Build history of the part. All positions in model axes, mm. Coordinates: 2 decimals unless noted, no trailing zeros. Write each loop counter-clockwise with the first axis right and the second up, starting at its lowest first coordinate (ties: lowest second). Pieces come first, ordered by that corner, then holes.
```python
from build123d import *

# Parameters (mm, degrees)
BASE_FLANGE1_DEPTH    = 76.2
CUT_EXTRUDE1_DEPTH    = 100.11903454
SKETCH4_R             = 8.334375
CUT_EXTRUDE2_DEPTH    = 100.669004783
FILLET1_R             = 9.525
FLAT_PATTERN1_START   = 4.7752
FLAT_PATTERN1_DEPTH   = 41.610875653
FLAT_PATTERN1_2_DEPTH = 4.7752
SKETCH6_R             = 4.9657
CUT_EXTRUDE4_DEPTH    = 89.346165933


# Read off the part's stored shape, not the designer's step: Flat-Pattern1
# Sheet-metal steps are written as plain solids
with BuildPart() as part:
    # Sketch1 → Base-Flange1 (new, symmetric)
    with BuildSketch(Plane(origin=(0, 0, 0), x_dir=(0, 0, -1), z_dir=(1, 0, 0))):
        with BuildLine():
            Line((0, 44.45), (0, 3.610410109))
            ThreePointArc((0, 3.610410109), (-0.932488229, 0.652935287), (-3.392675737, -1.234832983))
            Line((-3.392675737, -1.234832983), (-44.752861065, -16.288709326))
            Line((-44.752861065, -16.288709326), (-46.386075653, -11.801489123))
            Line((-46.386075653, -11.801489123), (-5.025890325, 3.25238722))
            ThreePointArc((-5.025890325, 3.25238722), (-4.844103071, 3.391877486), (-4.7752, 3.610410109))
            Line((-4.7752, 3.610410109), (-4.7752, 44.45))
            Line((-4.7752, 44.45), (0, 44.45))
        make_face()
    extrude(amount=BASE_FLANGE1_DEPTH, both=True)

    # Sketch3 → Cut-Extrude1 (cut, through all)
    with BuildSketch(Plane(origin=(0, -7.918276224, 35.717035898), x_dir=(1, 0, 0), z_dir=(0, -0.9396926207859093, -0.3420201433256664))):
        with BuildLine():
            Line((-76.2, -20.318857819), (-16.138866151, 7.766752504))
            ThreePointArc((-16.138866151, 7.766752504), (0, 11.353754961), (16.138866151, 7.766752504))
            Line((16.138866151, 7.766752504), (76.2, -20.318857819))
            Line((76.2, -20.318857819), (88.840930233, -20.318857819))
            Line((88.840930233, -20.318857819), (88.840930233, 63.227466393))
            Line((88.840930233, 63.227466393), (-88.840930233, 63.227466393))
            Line((-88.840930233, 63.227466393), (-88.840930233, -20.318857819))
            Line((-88.840930233, -20.318857819), (-76.2, -20.318857819))
        make_face()
    extrude(amount=CUT_EXTRUDE1_DEPTH, mode=Mode.SUBTRACT)

    # Sketch4 → Cut-Extrude2 (cut, through all)
    with BuildSketch(Plane.XY):
        with Locations(Location((50.8, 25.4, 0), (0, 0, 90))):
            Circle(SKETCH4_R)
        with Locations(Location((-50.8, 25.4, 0), (0, 0, 180))):
            Circle(SKETCH4_R)
    extrude(amount=CUT_EXTRUDE2_DEPTH, mode=Mode.SUBTRACT)

    # Fillet1
    fillet1_edges = [part.edges().sort_by_distance(p)[0] for p in [
        (76.2, 44.45, 2.3876),
        (-76.2, -3.212427662, 15.806947849),
        (76.2, -3.212427662, 15.806947849),
        (-76.2, 44.45, 2.3876),
    ]]
    fillet(fillet1_edges, radius=FILLET1_R)

    # Flat-Pattern1 outline → Flat-Pattern1 (cut)
    with BuildSketch(Plane.XY.offset(FLAT_PATTERN1_START)):
        with BuildLine():
            ThreePointArc((70.709716538, -14.097999428), (74.711053136, -10.58321022), (76.2, -5.469750042))
            Line((76.2, -5.469750042), (76.2, 5))
            Line((76.2, 5), (-76.2, 5))
            Line((-76.2, 5), (-76.2, -5.469750042))
            ThreePointArc((-76.2, -5.469750042), (-74.711053136, -10.58321022), (-70.709716538, -14.097999428))
            Line((-70.709716538, -14.097999428), (-16.138866151, -39.616259585))
            ThreePointArc((-16.138866151, -39.616259585), (0, -43.203262043), (16.138866151, -39.616259585))
            Line((16.138866151, -39.616259585), (70.709716538, -14.097999428))
        make_face()
    extrude(amount=FLAT_PATTERN1_DEPTH, mode=Mode.SUBTRACT)

    # Flat-Pattern1 2 outline → Flat-Pattern1 2 (add)
    with BuildSketch(Plane.XY):
        with BuildLine():
            ThreePointArc((70.709716538, -14.097999428), (74.711053136, -10.58321022), (76.2, -5.469750042))
            Line((76.2, -5.469750042), (76.2, 5))
            Line((76.2, 5), (-76.2, 5))
            Line((-76.2, 5), (-76.2, -5.469750042))
            ThreePointArc((-76.2, -5.469750042), (-74.711053136, -10.58321022), (-70.709716538, -14.097999428))
            Line((-70.709716538, -14.097999428), (-16.138866151, -39.616259585))
            ThreePointArc((-16.138866151, -39.616259585), (0, -43.203262043), (16.138866151, -39.616259585))
            Line((16.138866151, -39.616259585), (70.709716538, -14.097999428))
        make_face()
    extrude(amount=FLAT_PATTERN1_2_DEPTH)

    # Sketch6 → Cut-Extrude4 (cut, through all)
    with BuildSketch(Plane.XY.offset(4.7752)):
        with Locations((0, -28.575)):
            Circle(SKETCH6_R)
    extrude(amount=-CUT_EXTRUDE4_DEPTH, mode=Mode.SUBTRACT)


solid = part.part
```
1. Saw through at B-B on x = 0. List the corners of the cut face in (y, z), plus the area to 3 significant figures.
Computed values:
outline: (-43.2, 0) - (-33.54, 0) - (-33.54, 4.78) - (-43.2, 4.78) - close; (-23.61, 0) - (44.45, 0) - (44.45, 4.78) - (-23.61, 4.78) - close
area: 371 mm2
2. Flat gauge pin, fed straight in: pin 1 (1 mm diameter, centred on y = -15, z = 1, fed in from +X). Where does the tip first touch, or does it go through?
Computed values:
pin 1: stops at x = 69.85
3. Mould opens along Y. For faces 1 (the face through (-42.474, 25.034, 2.354)), 2 (the face through (-73.34, 41.73, 2.35)), 3 (the face through (76.2, 14, 2)), 4 (the face through (2.29, -32.98, 2.42)) say: +Y half, -Y half, draft (parallel to the pull), parting line (faces both ways), or undercut.
Computed values:
face 1: undercut
face 2: +Y half
face 3: draft
face 4: undercut
4. Probe line 1 along X through (y, z) = (25.4, 2.15); line 2 along X through (y, z) = (20, 2.2); line 3 along X through (y, z) = (-16, 3.6). List the from-to ranges inside material, lowest first.
Computed values:
line 1: x = -76.2 to -59.13, -42.47 to 42.47, 59.13 to 76.2
line 2: x = -76.2 to -57.15, -44.45 to 44.45, 57.15 to 76.2
line 3: x = -66.64 to 66.64
5. Saw through at C-C on z = 1.4. List the corners of the cut face in (x, y) (3 decimals).
Computed values:
outline: (-76.2, -5.47) arc R9.525 ccw to (-70.71, -14.098) - (-16.139, -39.616) arc R38.1 ccw to (16.139, -39.616) - (70.71, -14.098) arc R9.525 ccw to (76.2, -5.47) - (76.2, 34.925) arc R9.525 ccw to (66.675, 44.45) - (-66.675, 44.45) arc R9.525 ccw to (-76.2, 34.925) - close; hole circle Ø16.669 at (-50.8, 25.4); hole circle Ø9.931 at (0, -28.575); hole circle Ø16.669 at (50.8, 25.4)
6. Saw through at A-A on y = 25.4. List the corners of the cut face in (x, z), plus the area to 3 significant figures.
Computed values:
outline: (-76.2, 0) - (-59.13, 0) - (-59.13, 4.78) - (-76.2, 4.78) - close; (-42.47, 0) - (42.47, 0) - (42.47, 4.78) - (-42.47, 4.78) - close; (59.13, 0) - (76.2, 0) - (76.2, 4.78) - (59.13, 4.78) - close
area: 569 mm2
7. Saw through at D-D on x = -55. List the corners of the cut face in (y, z).
Computed values:
outline: (-21.44, 0) - (18.2, 0) - (18.2, 4.78) - (-21.44, 4.78) - close; (32.6, 0) - (44.45, 0) - (44.45, 4.78) - (32.6, 4.78) - close
